Geometry: see drawing. Coordinates: mm, zero at the bounding-box minimum. Round coordinates to 2 decimals unless told otherwise and drop trailing zeros. Write each loop counter-clockwise with the first axis right and the second up, starting at its lowest first coordinate (ties: lowest second). Pieces come first, ordered by that corner, then holes. Notation, with made-up numbers: M -3.5,61 L 27.5,61 A9 ccw 27.5,69 Z; hole C 74,5.5 d8. An arc over 180 degrees is marked long. Use a Markdown table: item, result.
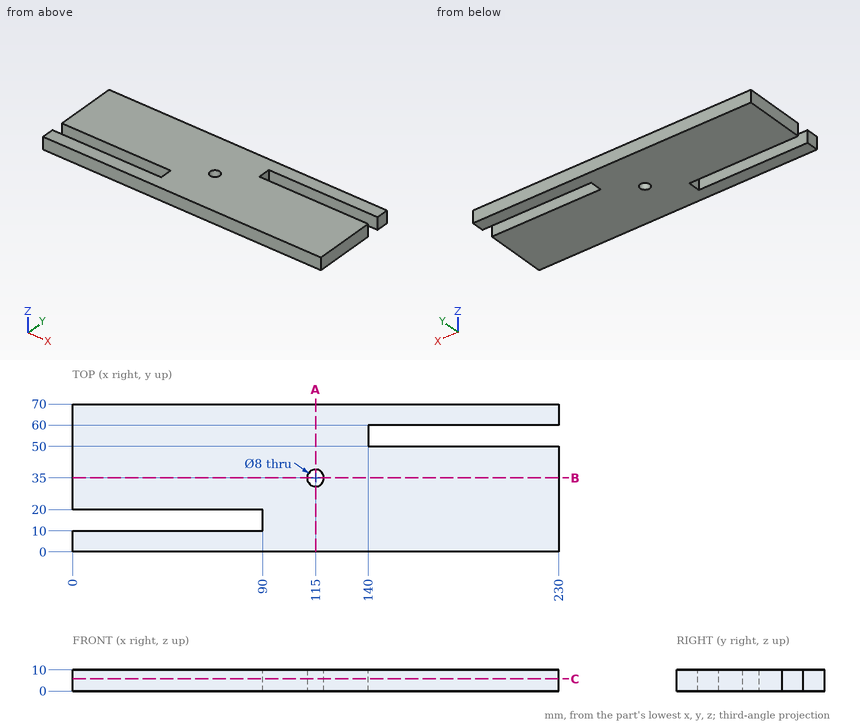
Q1. Line query: L1, parallel to Y at x = 159, z = 3.25; L2, parallel to Y at x = 115, z = 7.75; L3, parallel to X at y = 15.5, z = 2. Output: solid intervals per line, ascending.
Results are:
| item | result |
|---|---|
| L1 | 0 to 50, 60 to 70 |
| L2 | 0 to 31, 39 to 70 |
| L3 | 90 to 230 |
Q2. Section C-C on z = 5.75. Return loops of the section in (x, y), plus the area to 3 significant figures.
Results are:
| item | result |
|---|---|
| outline | M 0,0 L 230,0 L 230,50 L 140,50 L 140,60 L 230,60 L 230,70 L 0,70 L 0,20 L 90,20 L 90,10 L 0,10 Z; hole C 115,35 d8 |
| area | 14,200 mm^2 |
Q3. Section B-B on y = 35. Return loops of the section in (x, z).
Results are:
| item | result |
|---|---|
| outline | M 0,0 L 111,0 L 111,10 L 0,10 Z; M 119,0 L 230,0 L 230,10 L 119,10 Z |
Q4. First-contact query: pin 1 Ø6.5 at (x, y) = (115, 35) entering from +Z. Flat tip, straight axial feed; report the tip coordinate or a pass-through.
Results are:
| item | result |
|---|---|
| pin 1 | through |
Q5. Section A-A on x = 115. Return loops of the section in (y, z), plus the area to 3 significant figures.
Results are:
| item | result |
|---|---|
| outline | M 0,0 L 31,0 L 31,10 L 0,10 Z; M 39,0 L 70,0 L 70,10 L 39,10 Z |
| area | 620 mm^2 |
